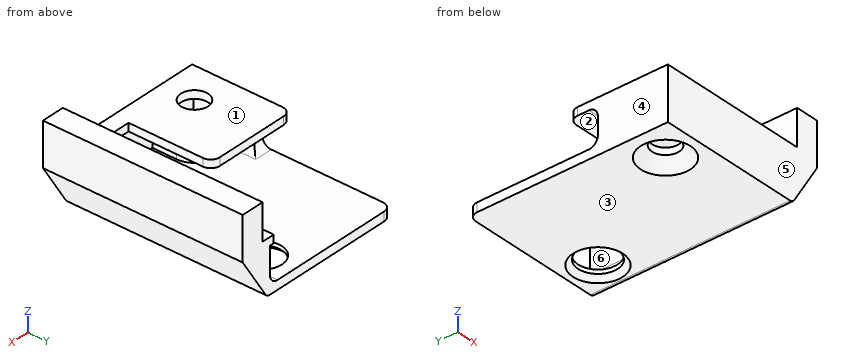
```python
from build123d import *

# Parameters (mm, degrees)
BOSS_EXTRUDE1_DEPTH                             = 15.4
CUT_EXTRUDE2_REACH                              = 25.918
SKETCH3_W                                       = 7.5
SKETCH3_H                                       = 11.5
BOSS_EXTRUDE3_REACH                             = 25.918
SKETCH4_W                                       = 0.8
SKETCH4_H                                       = 6.2
SKETCH4_W_2                                     = 2.8
SKETCH4_H_2                                     = 17.7
SKETCH10_W                                      = 4
SKETCH10_H                                      = 0.7
CUT_EXTRUDE4_DEPTH                              = 16.3
BOSS_EXTRUDE4_DEPTH                             = 0.8
CSK_FOR_M2_FLAT_HEAD_MACHINE_SCREW3_D           = 2.4
CSK_FOR_M2_FLAT_HEAD_MACHINE_SCREW3_CSINK_D     = 4.4
CSK_FOR_M2_FLAT_HEAD_MACHINE_SCREW3_CSINK_ANGLE = 90
MOVE_FACE1_BY                                   = 0.6
SKETCH14_W                                      = 8.2
SKETCH14_H                                      = 8.3
CUT_EXTRUDE6_DEPTH                              = 0.7
SKETCH3_2_W                                     = 7.5
SKETCH3_2_H                                     = 11.5
BOSS_EXTRUDE6_DEPTH                             = 0.8
FILLET3_R                                       = 0.8
CHAMFER1_SIZE                                   = 2.5
CHAMFER1_SIZE2                                  = 4
SKETCH12_W                                      = 2.0475
SKETCH12_H                                      = 3.18
BOSS_EXTRUDE5_DEPTH                             = 17.7
FILLET5_R                                       = 0.5
SKETCH11_R                                      = 1.75
CUT_EXTRUDE5_DEPTH                              = 25.492262043
CUT_EXTRUDE5_DIRECTION_2_REACH                  = 26.492


with BuildPart() as part:
    # Sketch2 → Boss-Extrude1 (new body)
    with BuildSketch(Plane(origin=(0, 0, 0), x_dir=(0, 0, -1), z_dir=(1, 0, 0))):
        Polygon((0, 0), (-4.65, 0), (-4.65, 17.7), (-3.85, 17.7), (-3.85, 0.8), (-0.7, 0.8), (-0.7, 17.7), (0, 17.7), align=None)
    extrude(amount=BOSS_EXTRUDE1_DEPTH)

    # Sketch3 → Cut-Extrude2 (cut, up to next)
    with BuildSketch(Plane.XY.offset(4.65), mode=Mode.PRIVATE) as cut_extrude2_sk1:
        with Locations((3.75, 11.95)):
            Rectangle(SKETCH3_W, SKETCH3_H)
    cut_extrude2_tool1 = extrude(cut_extrude2_sk1.sketch, amount=-CUT_EXTRUDE2_REACH, mode=Mode.PRIVATE) & part.part
    add(cut_extrude2_tool1.solids().sort_by_distance((3.75, 11.95, 4.65))[0], mode=Mode.SUBTRACT)

    # Sketch4 → Boss-Extrude3 (add, up to next)
    with BuildSketch(Plane.XY.offset(4.65), mode=Mode.PRIVATE) as boss_extrude3_sk1:
        with Locations((0.4, 3.1)):
            Rectangle(SKETCH4_W, SKETCH4_H)
    boss_extrude3_tool1 = extrude(boss_extrude3_sk1.sketch, amount=-BOSS_EXTRUDE3_REACH, mode=Mode.PRIVATE) - part.part
    # Sketch4 → Boss-Extrude3 (add, up to next)
    with BuildSketch(Plane.XY.offset(4.65), mode=Mode.PRIVATE) as boss_extrude3_sk2:
        with Locations((14, 8.85)):
            Rectangle(SKETCH4_W_2, SKETCH4_H_2)
    boss_extrude3_tool2 = extrude(boss_extrude3_sk2.sketch, amount=-BOSS_EXTRUDE3_REACH, mode=Mode.PRIVATE) - part.part
    add(boss_extrude3_tool1.solids().sort_by_distance((0.4, 3.1, 4.65))[0])
    add(boss_extrude3_tool2.solids().sort_by_distance((14, 8.85, 4.65))[0])

    # Sketch10 → Cut-Extrude4 (cut)
    with BuildSketch(Plane(origin=(0, 17.7, 0), x_dir=(1, 0, 0), z_dir=(0, 1, 0))):
        with Locations((10.2, -0.35)):
            Rectangle(SKETCH10_W, SKETCH10_H)
    extrude(amount=-CUT_EXTRUDE4_DEPTH, mode=Mode.SUBTRACT)

    # Sketch6 → Boss-Extrude4 (add)
    with BuildSketch(Plane(origin=(0, 0, 3.85), x_dir=(-1, 0, 0), z_dir=(0, 0, -1))):
        with BuildLine():
            Line((-0.8, 0.8), (-5.05, 0.8))
            Line((-5.05, 0.8), (-5.05, 2.95))
            ThreePointArc((-5.05, 2.95), (-4.508147545, 4.258147545), (-3.2, 4.8))
            Line((-3.2, 4.8), (-0.8, 4.8))
            Line((-0.8, 4.8), (-0.8, 0.8))
        make_face()
    extrude(amount=BOSS_EXTRUDE4_DEPTH)

    # CSK for M2 Flat Head Machine Screw3 (through all)
    with Locations(Plane(origin=(10.2, 14.95, 4.65), x_dir=(0, 1, 0), z_dir=(0, 0, 1))):
        with Locations((0, 0), (-12, 7)):
            CounterSinkHole(CSK_FOR_M2_FLAT_HEAD_MACHINE_SCREW3_D / 2, CSK_FOR_M2_FLAT_HEAD_MACHINE_SCREW3_CSINK_D / 2, counter_sink_angle=CSK_FOR_M2_FLAT_HEAD_MACHINE_SCREW3_CSINK_ANGLE)

    # Move Face1: a face moved inward by 0.6
    extrude(part.faces().sort_by_distance((4.1, 17.7, 0.35))[0], amount=MOVE_FACE1_BY, dir=(0, -1, 0), mode=Mode.SUBTRACT)

    # Sketch14 → Cut-Extrude6 (cut)
    with BuildSketch(Plane(origin=(0, 0, 0), x_dir=(-1, 0, 0), z_dir=(0, 0, -1))):
        with Locations((-4.1, 12.95)):
            Rectangle(SKETCH14_W, SKETCH14_H)
    extrude(amount=-CUT_EXTRUDE6_DEPTH, mode=Mode.SUBTRACT)

    # Sketch3<2> → Boss-Extrude6 (add)
    with BuildSketch(Plane.XY.offset(4.65)):
        with Locations((3.75, 11.95)):
            Rectangle(SKETCH3_2_W, SKETCH3_2_H)
    extrude(amount=-BOSS_EXTRUDE6_DEPTH)

    # Fillet3
    fillet3_edges = [part.edges().sort_by_distance(p)[0] for p in [
        (0.8, 5.5, 3.85),
        (0, 8.8, 0.35),
        (8.2, 8.8, 0.35),
        (0, 17.7, 4.25),
        (0.4, 6.2, 3.85),
        (0.4, 6.2, 0.7),
        (12.6, 9.25, 3.85),
    ]]
    fillet(fillet3_edges, radius=FILLET3_R)

    # Chamfer1
    chamfer1_edges = [part.edges().sort_by_distance(p)[0] for p in [
        (15.4, 8.85, 4.65),
    ]]
    chamfer1_side = [part.faces().sort_by_distance(p)[0] for p in [
        (7.829915164, 8.832514614, 4.65),
    ]]
    chamfer(chamfer1_edges, length=CHAMFER1_SIZE, length2=CHAMFER1_SIZE2, reference=chamfer1_side[0])

    # Sketch12 → Boss-Extrude5 (add)
    with BuildSketch(Plane(origin=(0, 17.7, 0), x_dir=(1, 0, 0), z_dir=(0, 1, 0))):
        with Locations((14.37625, 1.59)):
            Rectangle(SKETCH12_W, SKETCH12_H)
    extrude(amount=-BOSS_EXTRUDE5_DEPTH)

    # Fillet5
    fillet5_edges = [part.edges().sort_by_distance(p)[0] for p in [
        (12.9, 8.85, 4.65),
    ]]
    fillet(fillet5_edges, radius=FILLET5_R)

    # Sketch11 → Cut-Extrude5 (cut)
    with BuildSketch(Plane(origin=(0, 0, 3.85), x_dir=(-1, 0, 0), z_dir=(0, 0, -1))):
        with Locations(Location((-10.2, 14.95, 0), (0, 0, 270))):
            Circle(SKETCH11_R)
    extrude(amount=-CUT_EXTRUDE5_DEPTH, mode=Mode.SUBTRACT)

    # Sketch11 → Cut-Extrude5 direction 2 (cut, up to next)
    with BuildSketch(Plane(origin=(0, 0, 3.85), x_dir=(-1, 0, 0), z_dir=(0, 0, -1)), mode=Mode.PRIVATE) as cut_extrude5_direction_2_sk1:
        with Locations(Location((-10.2, 14.95, 0), (0, 0, 270))):
            Circle(SKETCH11_R)
    cut_extrude5_direction_2_tool1 = extrude(cut_extrude5_direction_2_sk1.sketch, amount=CUT_EXTRUDE5_DIRECTION_2_REACH, mode=Mode.PRIVATE) & part.part
    add(cut_extrude5_direction_2_tool1.solids().sort_by_distance((10.2, 14.95, 3.85))[0], mode=Mode.SUBTRACT)


with BuildPart() as body_2:
    # Mirror1: mirrored copy
    add(part.part.mirror(Plane(origin=(13.3525, 0, -3.18), x_dir=(1, 0, 0), z_dir=(0, 0, -1))))


solid = body_2.part
```
The listing builds one solid part. Answer for the finished solid, in the listing's coordinates (mm). Face numbers are marked on the shaded views. A direction names the side the tool comes from. Round coordinates to 2 decimals unless told otherwise and drop trailing zeros. Loops run counter-clockwise (first coordinate to the right, second up) from the corner with the lowest first, then second, coordinate; pieces in that order, holes last. Notation, with made-up numbers: (66, 87.25) -> (78, 87.25) arc R17 ccw to (78, 98.25) -> close; hole circle Ø7 at (66, 69). An arc over 180 degrees is marked (long way). Use one line per item in the form item = value.
1. The part is cut by section D-D on x = 6.5. Determine the outline of the cut face in (y, z), and give its area (3 significant figures).
Answer key:
outline = (0, -11.01) -> (17.7, -11.01) -> (17.7, -10.21) -> (0.8, -10.21) -> (0.8, -7.06) -> (8.8, -7.06) -> (8.8, -6.36) -> (0, -6.36) -> close
area = 22.8 mm²
2. The part is cut by section C-C on z = -6.75. Determine the outline of the cut face in (x, y), and give its area (3 significant figures).
Answer key:
outline = (0, 0) -> (15.4, 0) -> (15.4, 17.7) -> (12.2, 17.7) -> (12.2, 1.4) -> (8.2, 1.4) -> (8.2, 8) arc R0.8 ccw to (7.4, 8.8) -> (0.8, 8.8) arc R0.8 ccw to (0, 8) -> close; hole circle Ø2.4 at (3.2, 2.95)
area = 130 mm²
3. The part is cut by section A-A on x = 10.2. Determine the outline of the cut face in (y, z), and give its area (3 significant figures).
Answer key:
outline = (0, -11.01) -> (12.75, -11.01) -> (13.2, -10.56) -> (13.2, -10.21) -> (0.8, -10.21) -> (0.8, -7.06) -> (1.4, -7.06) -> (1.4, -6.36) -> (0, -6.36) -> close; (16.7, -10.56) -> (17.15, -11.01) -> (17.7, -11.01) -> (17.7, -10.21) -> (16.7, -10.21) -> close
area = 14.7 mm²
4. A tool of negligible diameter and unlimited length cuts with its end or side. For the marked faces 1, 2 and 3, from which of +Z, -Z, +X, -X, +Y, -Y can it reach the whole face along a straight path? Write none if from no direction.
Answer key:
face_1 = +Z, -X, +Y, -Y
face_2 = +Y
face_3 = -Z, +X, -X, +Y, -Y
5. For a pull along X with two mould halves and no side action, classify the marked faces 4, 5 and 6 as released by +X, released by -X, zero draft, split by the parting line, or undercut.
Answer key:
face_4 = released by -X
face_5 = zero draft
face_6 = undercut
6. Flat-ended cylindrical pins translate along their axes: pin 1 Ø0.9 at (x, z) = (1.5, -9.5) entering from +Y; pin 2 Ø0.9 at (x, z) = (0.5, -8.5) entering from +Y; pin 3 Ø2 at (x, z) = (7, -10) entering from -Y; pin 4 Ø3.5 at (y, z) = (10.5, -5.5) entering from -X. Find the tip coordinate at first contact, or state that the pin passes through.
Answer key:
pin_1 = 4.8
pin_2 = 6.2
pin_3 = 0
pin_4 = 12.2
7. Find the intervals of material crossed by probe 1 along Z at (x, y) = (7.5, 4.5); probe 2 along Y at (x, z) = (3.2, -6.55); probe 3 along Y at (x, z) = (3.2, -9.5), in increasing order. Write a range as [from, to].
Answer key:
probe_1 = [-11.01, -10.21], [-7.06, -6.36]
probe_2 = [0, 1.75], [4.15, 8.8]
probe_3 = [0, 1.75], [4.15, 4.8]
